```python
from build123d import *

# Parameters (mm, degrees)
CUT_EXTRUDE1_DEPTH   = 212.88306668
BOSS_EXTRUDE2_DEPTH  = 139.7
SKETCH9_R            = 35.95202499
BOSS_EXTRUDE3_DEPTH  = 4
CUT_EXTRUDE2_DEPTH   = 4
SKETCH11_W           = 10
SKETCH11_H           = 34
CUT_EXTRUDE3_DEPTH   = 15
RASPBERRY_PI_5_DEPTH = 5
GPS_SLOT_DEPTH       = 5.1
SKETCH14_W           = 12
SKETCH14_H           = 16
MPU_DEPTH            = 434.220724454
ALTIMETER_DEPTH      = 434.220724454
ALTIMETER_DEPTH_BACK = 3.54
SKETCH15_W           = 15.34
SKETCH15_H           = 20
SKETCH16_W           = 62.2
SKETCH16_H           = 25.5
PCA9685_DEPTH        = 2
SKETCH17_W           = 50
SKETCH17_H           = 27
ESP_32_1_DEPTH       = 5
SKETCH18_W           = 55
SKETCH18_H           = 30.1
BATTERY_1_DEPTH      = 3.5
SKETCH21_W           = 55
SKETCH21_H           = 30.1
BATTERY_2_DEPTH      = 3.5
SKETCH25_W           = 21.1
SKETCH25_H           = 43.1
STEP_DOWN_DEPTH      = 1
BOSS_EXTRUDE4_START  = -120
SKETCH27_R           = 36.3
SKETCH27_R_2         = 30
BOSS_EXTRUDE4_DEPTH  = 7
CUT_EXTRUDE4_START   = -127
SKETCH28_R           = 36.3
CUT_EXTRUDE4_DEPTH   = 480.865446219
SKETCH29_W           = 3.8
SKETCH29_H           = 24
BOSS_EXTRUDE5_DEPTH  = 5
SKETCH33_W           = 50
SKETCH33_H           = 27
ESP_32_2_DEPTH       = 5


with BuildPart() as part:
    # Sketch3 → Revolve1 (revolve)
    with BuildSketch(Plane.XY):
        with BuildLine():
            Line((285.74876522, 39.710021262), (285.74876522, 3.757996272))
            Line((285.74876522, 3.757996272), (80.74876522, 3.757996272))
            Line((80.74876522, 3.757996272), (80.74876522, 19.634316044))
            add(Edge.make_bspline(
                [(80.74876522, 19.634316044), (82.347112552, 19.950400666), (85.636412123, 20.593859316), (92.311794173, 21.870421625), (109.164486257, 24.943674568), (127.867996046, 27.977765645), (146.633052135, 30.604670801), (163.733801994, 32.658467989), (174.004488004, 33.801497199), (184.284802392, 34.855212792), (194.57611333, 35.797171826), (204.876878825, 36.627240946), (213.466527777, 37.244314669), (220.34120026, 37.693162367), (227.218898943, 38.097179671), (233.238636081, 38.411453209), (238.400481516, 38.652791264), (242.701722554, 38.8352093), (246.145182192, 38.969923968), (249.584994627, 39.093417446), (253.03241088, 39.20568842), (256.467961578, 39.306735697), (259.924132141, 39.396558203), (263.346991762, 39.475154984), (266.82565511, 39.542525204), (270.211898057, 39.598668148), (273.756466178, 39.643583219), (276.60509147, 39.673059099), (279.43950326, 39.691306197), (281.597603414, 39.703938851), (283.942998009, 39.708617629), (285.03032454, 39.710021262), (285.74876522, 39.710021262)],
                knots=[0.322773044, 0.322773044, 0.322773044, 0.322773044, 0.322773044, 0.341563488, 0.3614269, 0.401153715, 0.520334158, 0.56006097, 0.579924379, 0.599787787, 0.639514601, 0.679241414, 0.699104823, 0.718968231, 0.738831638, 0.758695045, 0.778558452, 0.788490156, 0.798421859, 0.808353563, 0.818285267, 0.828216971, 0.838148675, 0.848080378, 0.858012082, 0.867943786, 0.87787549, 0.887807193, 0.897738897, 0.902704749, 0.9076706, 0.917602304, 0.917602304, 0.917602304, 0.917602304, 0.917602304], degree=4))
        make_face()
    revolve(axis=Axis((285.74876522, 3.757996272, 0), (-1, 0, 0)))

    # Sketch6 → Cut-Extrude1 (cut, through all)
    with BuildSketch(Plane(origin=(285.74876522, 0, 0), x_dir=(0, 0, -1), z_dir=(1, 0, 0))):
        with BuildLine():
            Line((-5, -31.844645496), (-5, 39.36063804))
            ThreePointArc((-5, 39.360638041), (-35.95202499, 3.757996272), (-5, -31.844645496))
        make_face()
        with BuildLine():
            ThreePointArc((35.95202499, 3.757996272), (27.132160123, 27.346001444), (5, 39.36063804))
            Line((5, 39.36063804), (5, -31.844645496))
            ThreePointArc((5, -31.844645496), (27.132160123, -19.830008899), (35.95202499, 3.757996272))
        make_face()
    extrude(amount=-CUT_EXTRUDE1_DEPTH, mode=Mode.SUBTRACT)

    # Sketch8 → Boss-Extrude2 (add)
    with BuildSketch(Plane(origin=(285.74876522, 0, 0), x_dir=(0, 0, -1), z_dir=(1, 0, 0))):
        with BuildLine():
            Line((5, -31.844645496), (5, 39.360638041))
            ThreePointArc((5, 39.360638041), (0, 39.710021262), (-5, 39.360638041))
            Line((-5, 39.360638041), (-5, -31.844645496))
            ThreePointArc((-5, -31.844645496), (0, -32.194028718), (5, -31.844645496))
        make_face()
    extrude(amount=BOSS_EXTRUDE2_DEPTH)

    # Sketch9 → Boss-Extrude3 (add)
    with BuildSketch(Plane(origin=(425.44876522, 0, 0), x_dir=(0, 0, -1), z_dir=(1, 0, 0))):
        with Locations(Location((0, 3.757996272, 0), (0, 0, 262.00572083))):
            Circle(SKETCH9_R)
    extrude(amount=BOSS_EXTRUDE3_DEPTH)

    # Sketch10 → Cut-Extrude2 (cut)
    with BuildSketch(Plane(origin=(429.44876522, 0, 0), x_dir=(0, 0, -1), z_dir=(1, 0, 0))):
        Polygon((-17, -4.442003728), (-17, 11.957996272), (-8.2, 20.757996272), (8.2, 20.757996272), (17, 11.957996272), (17, -4.442003728), (8.2, -13.242003728), (-8.2, -13.242003728), align=None)
    extrude(amount=-CUT_EXTRUDE2_DEPTH, mode=Mode.SUBTRACT)

    # Sketch11 → Cut-Extrude3 (cut)
    with BuildSketch(Plane(origin=(425.44876522, 0, 0), x_dir=(0, 0, -1), z_dir=(1, 0, 0))):
        with Locations((0, 3.757996272)):
            Rectangle(SKETCH11_W, SKETCH11_H)
    extrude(amount=-CUT_EXTRUDE3_DEPTH, mode=Mode.SUBTRACT)

    # Sketch12 → Raspberry Pi 5 (cut)
    with BuildSketch(Plane.XY.offset(5)):
        with BuildLine():
            Line((404.44876522, -22.611276601), (321.44876522, -22.611276601))
            ThreePointArc((321.44876522, -22.611276601), (320.741658439, -22.318383382), (320.44876522, -21.611276601))
            Line((320.44876522, -21.611276601), (320.44876522, 32.388723399))
            ThreePointArc((320.44876522, 32.388723399), (320.741658439, 33.09583018), (321.44876522, 33.388723399))
            Line((321.44876522, 33.388723399), (404.44876522, 33.388723399))
            ThreePointArc((404.44876522, 33.388723399), (405.155872001, 33.09583018), (405.44876522, 32.388723399))
            Line((405.44876522, 32.388723399), (405.44876522, -21.611276601))
            ThreePointArc((405.44876522, -21.611276601), (405.155872001, -22.318383382), (404.44876522, -22.611276601))
        make_face()
    extrude(amount=-RASPBERRY_PI_5_DEPTH, mode=Mode.SUBTRACT)

    # Sketch13 → GPS Slot (cut)
    with BuildSketch(Plane.XY.offset(5)):
        with BuildLine():
            Line((202.636622216, 4.373367791), (169.986622216, 4.373367791))
            ThreePointArc((169.986622216, 4.373367791), (169.279515435, 4.666261009), (168.986622216, 5.373367791))
            Line((168.986622216, 5.373367791), (168.986622216, 28.973367791))
            ThreePointArc((168.986622216, 28.973367791), (169.279515435, 29.680474572), (169.986622216, 29.973367791))
            Line((169.986622216, 29.973367791), (202.636622216, 29.973367791))
            ThreePointArc((202.636622216, 29.973367791), (203.343728997, 29.680474572), (203.636622216, 28.973367791))
            Line((203.636622216, 28.973367791), (203.636622216, 5.373367791))
            ThreePointArc((203.636622216, 5.373367791), (203.343728997, 4.666261009), (202.636622216, 4.373367791))
        make_face()
    extrude(amount=-GPS_SLOT_DEPTH, mode=Mode.SUBTRACT)

    # Sketch14 → MPU (cut, through all)
    with BuildSketch(Plane.XY.offset(5)):
        with Locations((194.701703522, -9.951938862)):
            Rectangle(SKETCH14_W, SKETCH14_H)
    extrude(amount=-MPU_DEPTH, mode=Mode.SUBTRACT)

    # Sketch15 → Altimeter (cut, two sides: drawn at the far end of the back side and taken through both)
    with BuildSketch(Plane.XY.offset(5).offset(-ALTIMETER_DEPTH_BACK)):
        with Locations((176.990311954, -10.017213078)):
            Rectangle(SKETCH15_W, SKETCH15_H)
    extrude(amount=ALTIMETER_DEPTH + ALTIMETER_DEPTH_BACK, mode=Mode.SUBTRACT)

    # Sketch16 → PCA9685 (cut)
    with BuildSketch(Plane.XY.offset(5)):
        with Locations((117.775147159, 3.348372785)):
            Rectangle(SKETCH16_W, SKETCH16_H)
    extrude(amount=-PCA9685_DEPTH, mode=Mode.SUBTRACT)

    # Sketch17 → ESP-32 (1) (cut)
    with BuildSketch(Plane.XY.offset(5)):
        with Locations((233.414755785, -12.374476934)):
            Rectangle(SKETCH17_W, SKETCH17_H)
    extrude(amount=-ESP_32_1_DEPTH, mode=Mode.SUBTRACT)

    # Sketch18 → Battery 1 (cut)
    with BuildSketch(Plane(origin=(0, 0, -5), x_dir=(-1, 0, 0), z_dir=(0, 0, -1))):
        with Locations((-377.94876522, 19.967269146)):
            Rectangle(SKETCH18_W, SKETCH18_H)
    extrude(amount=-BATTERY_1_DEPTH, mode=Mode.SUBTRACT)

    # Sketch21 → Battery 2 (cut)
    with BuildSketch(Plane(origin=(0, 0, -5), x_dir=(-1, 0, 0), z_dir=(0, 0, -1))):
        with Locations((-377.94876522, -12.451276601)):
            Rectangle(SKETCH21_W, SKETCH21_H)
    extrude(amount=-BATTERY_2_DEPTH, mode=Mode.SUBTRACT)

    # Sketch25 → Step Down (cut)
    with BuildSketch(Plane(origin=(0, 0, -5), x_dir=(-1, 0, 0), z_dir=(0, 0, -1))):
        with Locations((-323.977591294, 5.876880331)):
            Rectangle(SKETCH25_W, SKETCH25_H)
    extrude(amount=-STEP_DOWN_DEPTH, mode=Mode.SUBTRACT)

    # Sketch27 → Boss-Extrude4 (add)
    with BuildSketch(Plane(origin=(429.44876522, 0, 0), x_dir=(0, 0, -1), z_dir=(1, 0, 0)).offset(BOSS_EXTRUDE4_START)):
        with Locations((0, 3.757996272)):
            Circle(SKETCH27_R)
        with Locations((0, 3.757996272)):
            Circle(SKETCH27_R_2, mode=Mode.SUBTRACT)
    extrude(amount=-BOSS_EXTRUDE4_DEPTH)

    # Sketch28 → Cut-Extrude4 (cut, through all)
    with BuildSketch(Plane(origin=(429.44876522, 0, 0), x_dir=(0, 0, -1), z_dir=(1, 0, 0)).offset(CUT_EXTRUDE4_START)):
        with Locations((0, 3.757996272)):
            Circle(SKETCH28_R)
    extrude(amount=CUT_EXTRUDE4_DEPTH, mode=Mode.SUBTRACT)

    # Sketch29 → Boss-Extrude5 (add)
    with BuildSketch(Plane(origin=(302.44876522, 0, 0), x_dir=(0, 0, -1), z_dir=(1, 0, 0))):
        with Locations((0, 3.757996272)):
            Rectangle(SKETCH29_W, SKETCH29_H)
    extrude(amount=BOSS_EXTRUDE5_DEPTH)

    # Sketch33 → ESP-32 (2) (cut)
    with BuildSketch(Plane.XY.offset(5)):
        with Locations((233.406186828, 18.864282523)):
            Rectangle(SKETCH33_W, SKETCH33_H)
    extrude(amount=-ESP_32_2_DEPTH, mode=Mode.SUBTRACT)


solid = part.part
```
Can you work these out from the model? Positions are in its coordinate system, mm. A direction names the side the tool comes from. Coordinates: 2 decimals unless noted, no trailing zeros. Loops run counter-clockwise (first coordinate to the right, second up) from the corner with the lowest first, then second, coordinate; pieces in that order, holes last. Notation, with made-up numbers: (7, 39.25) -> (59, 39.25) arc R18 ccw to (59, 62.25) -> close; hole circle Ø6 at (-19.5, -8.75). An arc over 180 degrees is marked (long way). Put each result on its own line as item: value. Start each with the question number.
Q1. For faces 4 (the face through (305, 4, -1.9)), 5 (the face through (305, 15.758, 0)), 6 (the face through (187, 4.373, 2)), which set-ups out of +Z, -Z, +X, -X, +Y, -Y let a thin tool reach every point of the face, with its end or its side?
Q2. Thinking about a two-plate mould opening in X: for faces 1 (the face through (293.98, 39.71, -0.07)), 2 (the face through (307.449, 4, 0)), 3 (the face through (258.406, 19, 3)), which applies, pulls with the +X half, pulls with the -X half, needs draft (parallel to the pull), parting line crosses it, or undercut?
Q3. I want a section at A-A (y = 12). Write out the boundary of the cut face in (x, z).
Q4. I'm going to push flat-ended pins straight in: P1, Ø4.5, axis at x = 176.5, y = -13, coming from the +Z side; P2, Ø4, axis at y = 24, z = 0, coming from the +X side; P3, Ø5, axis at x = 253, y = 24.5, coming from the +Z side. Where does each tip first touch, or does it pass through?
Q5. If I drill on line 1 (X direction, y = -7.5, z = 3.75); line 2 (X direction, y = -11.5, z = 4.25); line 3 (X direction, y = 16.5, z = 0.5), over which ranges is the centre line in solid material (lowest first)? Write a range as [from, to].
Taken from the geometry:
1. face 4: -Z, +X, +Y, -Y
1. face 5: +Z, -Z, +X, +Y
1. face 6: +Z
2. face 1: needs draft
2. face 2: pulls with the +X half
2. face 3: undercut
3. outline: (80.75, -5) -> (302.45, -5) -> (302.45, -1.9) -> (307.45, -1.9) -> (307.45, 1.9) -> (302.45, 1.9) -> (302.45, 5) -> (258.41, 5) -> (258.41, 0) -> (208.41, 0) -> (208.41, 5) -> (203.64, 5) -> (203.64, -0.1) -> (168.99, -0.1) -> (168.99, 5) -> (148.88, 5) -> (148.88, 3) -> (86.68, 3) -> (86.68, 5) -> (80.75, 5) -> close
4. P1: stops at z = 1.46
4. P2: stops at x = 302.45
4. P3: stops at z = 0
5. line 1: x = [80.75, 86.68], [148.88, 169.32], [184.66, 188.7], [200.7, 208.41], [258.41, 302.45]
5. line 2: x = [80.75, 169.32], [184.66, 188.7], [200.7, 208.41], [258.41, 302.45]
5. line 3: x = [80.75, 168.99], [203.64, 208.41], [258.41, 302.45]
